Model file for the job. Use its own axes, mm. Face numbers are marked on the shaded views. A direction names the side the tool comes from. Coordinates: 2 decimals unless noted, no trailing zeros. Loops run counter-clockwise (first coordinate to the right, second up) from the corner with the lowest first, then second, coordinate; pieces in that order, holes last.
Autodesk Inventor part; units mm, degrees
ref_plane "YZ Plane" through (0, 0, 0) normal (1, 0, 0) x (0, 1, 0)
ref_plane "XZ Plane" through (0, 0, 0) normal (0, 1, 0) x (-1, 0, 0)
ref_plane "XY Plane" through (0, 0, 0) normal (0, 0, 1) x (1, 0, 0)
sketch "スケッチ1" plane through (0, 0, 0) normal (0, 0, 1) x (1, 0, 0)
  line L0 (0, 0) -> (0, 3.5)
  line L1 (0, 3.5) -> (0, 3.5)
  line L2 (0, 3.5) -> (0, 8)
  line L3 (0, 8) -> (6.3, 8)
  line L4 (6.3, 8) -> (6.3, 3)
  line L5 (6.3, 3) -> (3.8, 3)
  line L6 (3.8, 3) -> (3.8, 0)
  line L7 (3.8, 0) -> (0, 0)
  dimension "d0" = 3.5
  dimension "d1" = 3
  dimension "d2" = 2.5
  dimension "d4" = 0
  dimension "d5" = 8
  dimension "d34" = 3.8
revolve "回転1" add sketch "スケッチ1" angle 360 about axis through (3.8, 0, 0) along (-1, 0, 0)
sketch "スケッチ2" plane through (6.3, 0, 0) normal (1, 0, 0) x (0, 0, -1)
  point P0 (0, 0)
  point P1 (-5.5, 0)
  point P2 (5.5, 0)
  dimension "d10" = 5.5
  dimension "d11" = 5.5
hole "穴1" at (6.3, 0, 5.5) at (6.3, 0, -5.5) direction (-1, 0, 0) diameter 2.9 end through all counterbore diameter 5.5 counterbore depth 2.5
chamfer "面取り5" distance 0.5 angle 45 2 edges at (6.3, 3, 0) (6.3, -3, 0)
fillet "フィレット2" radius 0.5 8 edges at (4.8, 0.8377, -2.8807) (4.8, 0.8377, 2.8807) (4.8, -0.8377, 2.8807) (4.8, -0.8377, -2.8807) (5.05, 1.3765, -7.8807) (5.05, 1.3765, 7.8807) (5.05, -1.3765, 7.8807) (5.05, -1.3765, -7.8807)
properties part number "unit-base4" material "ABS プラスチック"
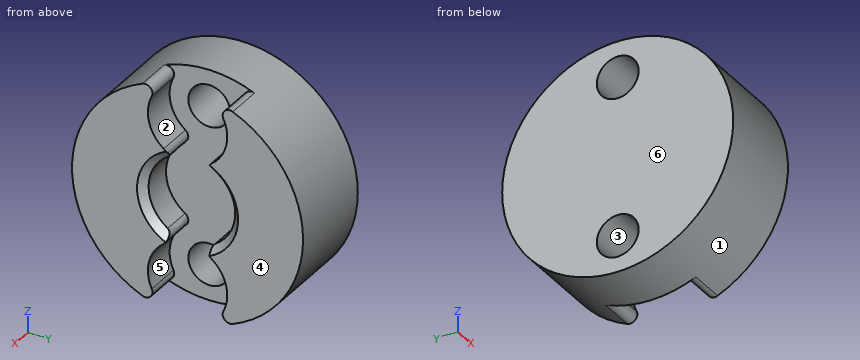
Q1. Slice it at A-A (z = 5.5). List the corners of the cut face in (x, y).
Answers:
outline: (0, -5.81) - (6.3, -5.81) - (6.3, -2.75) - (3.8, -2.75) - (3.8, -1.45) - (0, -1.45) - close; (0, 1.45) - (3.8, 1.45) - (3.8, 2.75) - (6.3, 2.75) - (6.3, 5.81) - (0, 5.81) - close
Q2. Slice it at B-B (y = 0.25). List the corners of the cut face in (x, z).
Answers:
outline: (0, -8) - (3.8, -8) - (3.8, -6.93) - (0, -6.93) - close; (0, -4.07) - (3.8, -4.07) - (3.8, 4.07) - (0, 4.07) - close; (0, 6.93) - (3.8, 6.93) - (3.8, 8) - (0, 8) - close
Q3. Flat gauge pins, fed straight in: P1, Ø1.5, axis at x = 5.5, y = -0.5, coming from the +Z side; P2, Ø4, axis at y = 0, z = -5.5, coming from the +X side. Where does each tip first touch, or does it go through?
Answers:
P1: passes through
P2: stops at x = 3.8
Q4. Which spindle directions (+Z, -Z, +X, -X, +Y, -Y) get a long thin tool onto all of the face, cutting with end or side? Do the marked faces 5 and 6. Say none if no direction does.
Answers:
face 5: +X
face 6: +Z, -Z, -X, +Y, -Y
Q5. Slice it at D-D (x = 3.5). List the corners of the cut face in (y, z), and give its area (3 significant figures).
Answers:
outline: circle Ø16 at (0, 0); hole circle Ø2.9 at (0, -5.5); hole circle Ø2.9 at (0, 5.5)
area: 188 mm2
Q6. Drill centre lines: line 1 (Z direction, x = 2.35, y = 0); line 2 (X direction, y = -0.25, z = 7); line 3 (Z direction, x = 2.5, y = -1.25). Where is each one in solid material? Low to high.
Answers:
line 1: z = -8 to -6.95, -4.05 to 4.05, 6.95 to 8
line 2: x = 0 to 3.8
line 3: z = -7.9 to -6.23, -4.77 to 4.77, 6.23 to 7.9
Q7. Mould opens along Y. For the marked faces 1, 2, 3 and 4 say: +Y half, -Y half, draft (parallel to the pull), parting line (faces both ways), or undercut.
Answers:
face 1: parting line
face 2: undercut
face 3: undercut
face 4: draft
Q8. Slice it at C-C (z = 0). List the corners of the cut face in (x, y).
Answers:
outline: (0, -8) - (6.3, -8) - (6.3, -3.5) - (5.8, -3) - (3.8, -3) - (3.8, 3) - (5.8, 3) - (6.3, 3.5) - (6.3, 8) - (0, 8) - close
